Work out the finished part from the listing and answer in its coordinate system (mm). Face numbers are marked on the shaded views. A direction names the side the tool comes from. Coordinates: 2 decimals unless noted, no trailing zeros. Order: outer loops, then holes, each group sorted by start corner. A loop starts at its lowest first (then second) coordinate and runs counter-clockwise, first axis right, second up. Notation, with made-up numbers: M 88,39.5 L 133,39.5 A30 ccw 133,68.5 Z; hole C 60,-9 d4. An arc over 180 degrees is marked long. Answer in a Markdown table with one row per item. Add a question column.
Item 1: Consider line 1 (Y direction, x = -25, z = 5.25); line 2 (Y direction, x = 39.5, z = 6.5); line 3 (X direction, y = -3.5, z = -0.75). Determine where each line is inside the solid, lowest interval first. Write a range as from..to.
Item 2: The mould has two halves that part along X. Classify the marked faces 1 and 2: released by +X, released by -X, zero draft, split by the parting line, or undercut.
Item 3: The part is cut by section C-C (z = 1.5). Write down the section's boundary in (x, y).
Item 4: Which of the six approach directions +Z, -Z, +X, -X, +Y, -Y give full straight-line access (tool end or side, diameter ignored) to the marked faces 3, 4 and 5?
Item 5: The part is cut by section B-B (x = 48). Write down the section's boundary in (y, z), then the cut area to 3 significant figures.
Item 6: Flat-ended cylindrical pins translate along their axes: pin 1 Ø1.5 at (x, y) = (-16, 0.5) entering from +Z; pin 2 Ø6 at (x, y) = (12.5, 3) entering from -Z; pin 3 Ø3 at (y, z) = (-0.5, 2) entering from +X. Find the tip coordinate at first contact, or state that the pin passes through.
Item 7: The part is cut by section A-A (y = 0). Write down the section's boundary in (x, z).
from build123d import *

# Parameters (mm, degrees)
F1_DEPTH  = 6
F3_DEPTH  = 3
F4_R      = 2.5
F5_W      = 5
F5_H      = 30.1
F6_DEPTH  = 1.25
F8_DEPTH  = 6
F10_DEPTH = 3
F11_R     = 2
F12_R     = 0.54999


# Not quite as in the source:
# - a fillet or chamfer is up to 0.001 mm smaller than in the source, because OpenCascade refuses the exact size


with BuildPart() as f1:
    # F0 (on Top) → F1 (new body)
    with BuildSketch(Plane.XY):
        with BuildLine():
            Line((49.5, 14.5), (-49.5, 14.5))
            ThreePointArc((-49.5, 14.5), (-64, 0), (-49.5, -14.5))
            Line((-49.5, -14.5), (49.5, -14.5))
            ThreePointArc((49.5, -14.5), (64, 0), (49.5, 14.5))
        make_face()
    extrude(amount=F1_DEPTH)

    # F2 (on face) → F3 (join)
    with BuildSketch(Plane.XY.offset(6)):
        with BuildLine():
            Line((50, 19.5), (-50, 19.5))
            ThreePointArc((-50, 19.5), (-69.5, 0), (-50, -19.5))
            Line((-50, -19.5), (50, -19.5))
            ThreePointArc((50, -19.5), (69.5, 0), (50, 19.5))
        make_face()
    extrude(amount=F3_DEPTH)

    # F4
    f4_edges = [f1.edges().sort_by_distance(p)[0] for p in [
        (0, -19.5, 9),
    ]]
    fillet(f4_edges, radius=F4_R)

    # F5 (on face) → F6 (join)
    with BuildSketch(Plane(origin=(0, 0, 0), x_dir=(1, 0, 0), z_dir=(0, 0, -1))):
        with Locations((-42, 0)):
            Rectangle(F5_W, F5_H)
        with Locations((42, 0)):
            Rectangle(F5_W, F5_H)
    extrude(amount=F6_DEPTH)

    # F7 (on face) → F8 (cut)
    with BuildSketch(Plane.XY.offset(9)):
        with BuildLine():
            Line((50, 10), (-50, 10))
            ThreePointArc((-50, 10), (-60, 0), (-50, -10))
            Line((-50, -10), (50, -10))
            ThreePointArc((50, -10), (60, 0), (50, 10))
        make_face()
    extrude(amount=-F8_DEPTH, mode=Mode.SUBTRACT)

    # F9 (on face) → F10 (join)
    with BuildSketch(Plane.XY.offset(9)):
        with BuildLine():
            Line((50, 10), (-50, 10))
            ThreePointArc((-50, 10), (-60, 0), (-50, -10))
            Line((-50, -10), (50, -10))
            ThreePointArc((50, -10), (60, 0), (50, 10))
        make_face()
        with BuildLine():
            ThreePointArc((50, 7), (57, 0), (50, -7))
            Line((50, -7), (-50, -7))
            ThreePointArc((-50, -7), (-57, 0), (-50, 7))
            Line((-50, 7), (50, 7))
        make_face(mode=Mode.SUBTRACT)
    extrude(amount=-F10_DEPTH)

    # F11
    f11_edges = [f1.edges().sort_by_distance(p)[0] for p in [
        (0, 7, 9),
    ]]
    fillet(f11_edges, radius=F11_R)

    # F12 (radius 0.55 in the source; OpenCascade refuses exactly that, so slightly less here)
    f12_edges = [f1.edges().sort_by_distance(p)[0] for p in [
        (-42, -15.05, 0),
        (-42, -15.05, -1.25),
        (42, -15.05, -1.25),
        (42, -15.05, 0),
        (-42, 15.05, -1.25),
        (-42, 15.05, 0),
        (42, 15.05, 0),
        (42, 15.05, -1.25),
    ]]
    fillet(f12_edges, radius=F12_R)


solid = f1.part
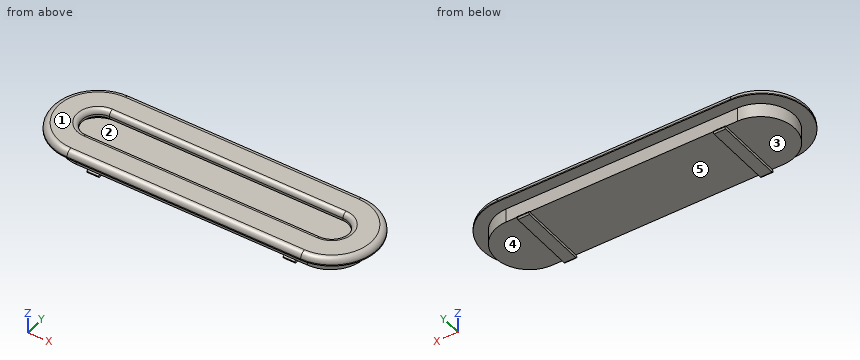
Reply:
| question | item | result |
|---|---|---|
| 1 | line 1 | y = -14.5..-10, 10..14.5 |
| 1 | line 2 | y = -19.5..-7, 7..19.5 |
| 1 | line 3 | x = -44.5..-39.5, 39.5..44.5 |
| 2 | face 1 | zero draft |
| 2 | face 2 | undercut |
| 3 | outline | M -49.5,-14.5 L 49.5,-14.5 A14.5 ccw 49.5,14.5 L -49.5,14.5 A14.5 ccw Z |
| 4 | face 3 | -Z, -X, +Y, -Y |
| 4 | face 4 | -Z, +X, +Y, -Y |
| 4 | face 5 | -Z, +Y, -Y |
| 5 | outline | M -19.5,6 L -14.5,6 L -14.5,0 L 14.5,0 L 14.5,6 L 19.5,6 L 19.5,6.5 A2.5 ccw 17,9 L 9,9 A2 ccw 7,7 L 7,6 L 10,6 L 10,3 L -10,3 L -10,6 L -7,6 L -7,7 A2 ccw -9,9 L -17,9 A2.5 ccw -19.5,6.5 Z |
| 5 | area | 185 mm2 |
| 6 | pin 1 | stops at z = 3 |
| 6 | pin 2 | stops at z = 0 |
| 6 | pin 3 | stops at x = 64 |
| 7 | outline | M -69.5,6 L -64,6 L -64,0 L -44.5,0 L -44.5,-1.25 L -39.5,-1.25 L -39.5,0 L 39.5,0 L 39.5,-1.25 L 44.5,-1.25 L 44.5,0 L 64,0 L 64,6 L 69.5,6 L 69.5,6.5 A2.5 ccw 67,9 L 59,9 A2 ccw 57,7 L 57,6 L 60,6 L 60,3 L -60,3 L -60,6 L -57,6 L -57,7 A2 ccw -59,9 L -67,9 A2.5 ccw -69.5,6.5 Z |
